For this review, take the finished solid that the model builds, in its own axes (mm). Face numbers are marked on the shaded views. A direction names the side the tool comes from. Round coordinates to 2 decimals unless told otherwise and drop trailing zeros. Order: outer loops, then holes, each group sorted by start corner. A loop starts at its lowest first (then second) coordinate and runs counter-clockwise, first axis right, second up. Notation, with made-up numbers: (-25.5, 35.5) - (15.5, 35.5) arc R25 ccw to (15.5, 47.5) - close; hole circle Ø1 at (13.25, -6.5). An arc over 180 degrees is marked (long way). Write each question's results on one line, items separated by ' | '. Start each with the question number.
(1) Take a section at B-B, the plane z = 34.5. Give the boundary of the cut face in (x, y).
(2) Take a section at C-C, the plane y = -6. Give the boundary of the cut face in (x, z).
(3) Take a section at A-A, the plane x = 11.5. Give the boundary of the cut face in (y, z), plus the area to 3 significant figures.
(4) For the marked faces 4, 5 and 6, list the 3-axis set-ups (+Z, -Z, +X, -X, +Y, -Y) from which the entire face can be reached by the end or side of a thin tool; tool diameter is ignored.
(5) Insertion check: pin 1 Ø3 at (x, y) = (7.5, 3.5) entering from -Z; pin 2 Ø9 at (x, y) = (11, -20.5) entering from -Z; pin 3 Ø4 at (x, y) = (6.5, 9) entering from +Z. Each pin has a flat end and moves straight along its axis. Give the tip position at first contact, or say it passes through.
(6) For L1, parallel to X at y = -24.5, z = 34.5; L2, parallel to Y at x = 7, z = 29; L3, parallel to Y at x = 9.25, z = 35, list the stretches that pass through material, from the lowest coordinate up. Write a range as from..to.
(7) Take a section at D-D, the plane x = 15.75. Give the boundary of the cut face in (y, z).
(8) Draft analysis for pull direction Z (two halves, no side actions). For the marked faces 1, 2 and 3, state which applies: pulls with the +Z half, pulls with the -Z half, needs draft (parallel to the pull), parting line crosses it, or undercut.
```python
from build123d import *

# Parameters (mm, degrees)
F0_W     = 50.8
F0_H     = 7.62
F1_DEPTH = 17.78
F3_DEPTH = 25.4
F4_W     = 10.16
F4_H     = 3.81
F5_DEPTH = 38.1
F4_R     = 1.27
F6_DEPTH = 7.62


with BuildPart() as f1:
    # F0 (on Right) → F1 (new body)
    with BuildSketch(Plane.YZ):
        with Locations((-19.6553, 37.308002)):
            Rectangle(F0_W, F0_H)
        Polygon((13.3647, 41.118002), (5.7447, 41.118002), (5.7447, 33.498002), (5.7447, 25.878002), (13.3647, 25.878002), align=None)
    extrude(amount=F1_DEPTH)

    # F2 (on face) → F3 (cut)
    with BuildSketch(Plane.YZ.offset(17.78)):
        with BuildLine():
            ThreePointArc((-45.0553, 35.032712), (-16.00334, 39.592575), (13.3647, 41.118002))
            Line((13.3647, 41.118002), (-45.0553, 41.118002))
            Line((-45.0553, 41.118002), (-45.0553, 35.032712))
        make_face()
    extrude(amount=-F3_DEPTH, mode=Mode.SUBTRACT)

    # F4 (on face) → F5 (cut)
    with BuildSketch(Plane(origin=(0, 13.3647, 0), x_dir=(-1, 0, 0), z_dir=(0, 1, 0))):
        with Locations((-8.89, 35.403002)):
            Rectangle(F4_W, F4_H)
    extrude(amount=-F5_DEPTH, mode=Mode.SUBTRACT)

    # F4 (on face) → F6 (cut)
    with BuildSketch(Plane(origin=(0, 13.3647, 0), x_dir=(-1, 0, 0), z_dir=(0, 1, 0))):
        with Locations((-1.905, 37.308002)):
            Circle(F4_R)
        with Locations((-15.875, 37.308002)):
            Circle(F4_R)
    extrude(amount=-F6_DEPTH, mode=Mode.SUBTRACT)


solid = f1.part
```
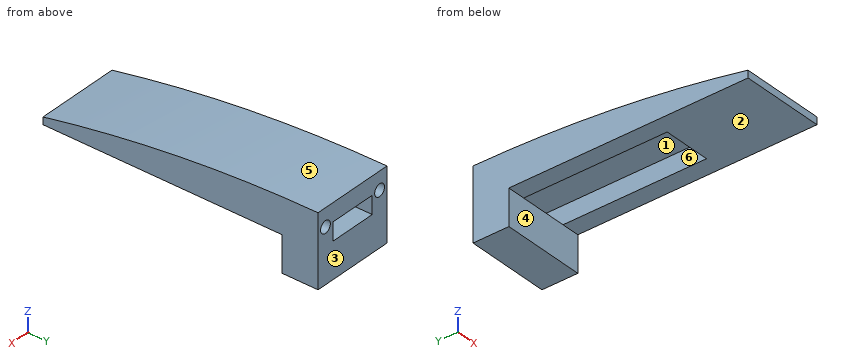
Results below:
1) outline: (0, -45.06) - (17.78, -45.06) - (17.78, 13.36) - (13.97, 13.36) - (13.97, -24.74) - (3.81, -24.74) - (3.81, 13.36) - (0, 13.36) - close
2) outline: (0, 33.5) - (3.81, 33.5) - (3.81, 37.31) - (13.97, 37.31) - (13.97, 33.5) - (17.78, 33.5) - (17.78, 40.46) - (0, 40.46) - close
3) outline: (-45.06, 33.5) - (-24.74, 33.5) - (-24.74, 37.31) - (13.36, 37.31) - (13.36, 41.12) arc R283.46 ccw to (-45.06, 35.03) - close; (5.74, 25.88) - (13.36, 25.88) - (13.36, 33.5) - (5.74, 33.5) - close | area: 240 mm^2
4) face 4: -Z, +X, -X, -Y | face 5: +Z, +X, -X, -Y | face 6: +Y
5) pin 1: stops at z = 37.31 | pin 2: stops at z = 33.5 | pin 3: stops at z = 41.11
6) L1: x = 0..3.81, 13.97..17.78 | L2: y = 5.74..13.36 | L3: y = -45.06..-24.74
7) outline: (-45.06, 33.5) - (5.74, 33.5) - (5.74, 25.88) - (13.36, 25.88) - (13.36, 36.04) - (5.74, 36.04) - (5.74, 38.57) - (13.36, 38.57) - (13.36, 41.12) arc R283.46 ccw to (-45.06, 35.03) - close
8) face 1: undercut | face 2: pulls with the -Z half | face 3: needs draft
